Could you check a few things on this model? Use its own coordinates, in mm. A direction names the side the tool comes from. Coordinates: 2 decimals unless noted, no trailing zeros. Write each loop counter-clockwise with the first axis right and the second up, starting at its lowest first coordinate (ties: lowest second). Pieces come first, ordered by that corner, then holes. Notation, with made-up numbers: M 28.5,-16 L 45.5,-16 A25 cw 45.5,18 Z; hole C -2,-3.75 d6. An arc over 180 degrees is marked long. Write item = value, one per line.
```python
from build123d import *

# Parameters (mm, degrees)
F0_R     = 11.0236
F1_DEPTH = 6.35


with BuildPart() as f1:
    # F0 (on Front) → F1 (new body)
    with BuildSketch(Plane.XZ):
        with BuildLine():
            ThreePointArc((0.3274680596, -14.2837467396), (10.2179096725, -9.9863395783), (14.2875, 0))
            ThreePointArc((14.2875, 0), (13.8765823163, 3.4019287867), (12.6674657785, 6.6081742563))
            ThreePointArc((12.6674657785, 6.6081742563), (12.3386048381, 7.157527699), (12.0249856082, 7.7157227382))
            ThreePointArc((12.0249856082, 7.7157227382), (-0.0794118424, 14.2872793075), (-12.1100113559, 7.581575114))
            ThreePointArc((-12.1100113559, 7.581575114), (-12.3736819292, 7.1101281538), (-12.6482244827, 6.6449284184))
            ThreePointArc((-12.6482244827, 6.6449284184), (-12.2974900055, -7.2735408032), (-0.2689126433, -14.2849691018))
            ThreePointArc((-0.2689126433, -14.2849691018), (0.0292737936, -14.2824480224), (0.3274680596, -14.2837467396))
        make_face()
        Circle(F0_R, mode=Mode.SUBTRACT)
        with BuildLine():
            ThreePointArc((12.6674657785, 6.6081742563), (13.8765823163, 3.4019287867), (14.2875, 0))
            ThreePointArc((14.2875, 0), (10.2179096725, -9.9863395783), (0.3274680596, -14.2837467396))
            ThreePointArc((0.3274680596, -14.2837467396), (10.9182683676, -16.9609416049), (19.1217645686, -24.1744756619))
            Line((19.1217645686, -24.1744756619), (14.2986624039, -15.99905024))
            Line((14.2986624039, -15.99905024), (20.7900538279, -4.5075300019))
            Line((20.7900538279, -4.5075300019), (31.3741279928, -4.4080458119))
            ThreePointArc((31.3741279928, -4.4080458119), (20.6570695125, -1.2156835719), (12.6674657785, 6.6081742563))
        make_face()
        with BuildLine():
            ThreePointArc((12.0249856082, 7.7157227382), (12.3386048381, 7.157527699), (12.6674657785, 6.6081742563))
            ThreePointArc((12.6674657785, 6.6081742563), (12.3586388725, 7.1691492849), (12.0249856082, 7.7157227382))
        make_face()
        with BuildLine():
            ThreePointArc((-0.2689126433, -14.2849691018), (0.0292840868, -14.2874699892), (0.3274680596, -14.2837467396))
            ThreePointArc((0.3274680596, -14.2837467396), (0.0292737936, -14.2824480224), (-0.2689126433, -14.2849691018))
        make_face()
        with BuildLine():
            ThreePointArc((-12.1100113559, 7.581575114), (-0.0794118424, 14.2872793075), (12.0249856082, 7.7157227382))
            ThreePointArc((12.0249856082, 7.7157227382), (9.2100112148, 18.0768557667), (11.3474304636, 28.5986710771))
            Line((11.3474304636, 28.5986710771), (6.7062527423, 20.3825300019))
            Line((6.7062527423, 20.3825300019), (-6.4913914239, 20.258479762))
            Line((-6.4913914239, 20.258479762), (-11.8801477461, 29.3927203242))
            ThreePointArc((-11.8801477461, 29.3927203242), (-9.2812144735, 18.4585467989), (-12.1100113559, 7.581575114))
        make_face()
        with BuildLine():
            ThreePointArc((33.9876979941, -4.383479762), (32.6812582501, -4.4324944701), (31.3741279928, -4.4080458119))
            Line((31.3741279928, -4.4080458119), (20.7900538279, -4.5075300019))
            Line((20.7900538279, -4.5075300019), (14.2986624039, -15.99905024))
            Line((14.2986624039, -15.99905024), (19.1217645686, -24.1744756619))
            ThreePointArc((19.1217645686, -24.1744756619), (20.1269642499, -25.7329626623), (21.0049151462, -27.366520238))
            Line((21.0049151462, -27.366520238), (34.2025593124, -27.2424699981))
            Line((34.2025593124, -27.2424699981), (40.6939507364, -15.75094976))
            Line((40.6939507364, -15.75094976), (33.9876979941, -4.383479762))
        make_face()
        Polygon((22.5339984594, -24.6596288042), (17.4074408075, -15.9698295168), (22.3697489183, -7.1852007126), (32.4586146809, -7.0903711958), (37.5851723328, -15.7801704832), (32.622864222, -24.5647992874), align=None, mode=Mode.SUBTRACT)
        with BuildLine():
            Line((33.9876979941, -4.383479762), (31.3741279928, -4.4080458119))
            ThreePointArc((31.3741279928, -4.4080458119), (32.6812582501, -4.4324944701), (33.9876979941, -4.383479762))
        make_face()
        with BuildLine():
            ThreePointArc((-19.5323350277, -25.0159672189), (-11.251794814, -17.2249549892), (-0.2689126433, -14.2849691018))
            ThreePointArc((-0.2689126433, -14.2849691018), (-12.2974900055, -7.2735408032), (-12.6482244827, 6.6449284184))
            ThreePointArc((-12.6482244827, 6.6449284184), (-20.2295725455, -1.03712802), (-30.4613844896, -4.4723651173))
            Line((-30.4613844896, -4.4723651173), (-21.0049151462, -4.383479762))
            Line((-21.0049151462, -4.383479762), (-14.2986624039, -15.75094976))
            Line((-14.2986624039, -15.75094976), (-19.5323350277, -25.0159672189))
        make_face()
        with BuildLine():
            ThreePointArc((21.0049151462, -27.366520238), (20.1269642499, -25.7329626623), (19.1217645686, -24.1744756619))
            Line((19.1217645686, -24.1744756619), (21.0049151462, -27.366520238))
        make_face()
        with BuildLine():
            ThreePointArc((-12.6482244827, 6.6449284184), (-12.3736819292, 7.1101281538), (-12.1100113559, 7.581575114))
            ThreePointArc((-12.1100113559, 7.581575114), (-12.3879734912, 7.1183403285), (-12.6482244827, 6.6449284184))
        make_face()
        with BuildLine():
            ThreePointArc((13.1976441662, 31.87405024), (12.2062266956, 30.2738185559), (11.3474304636, 28.5986710771))
            Line((11.3474304636, 28.5986710771), (13.1976441662, 31.87405024))
        make_face()
        with BuildLine():
            Line((6.7062527423, 20.3825300019), (11.3474304636, 28.5986710771))
            ThreePointArc((11.3474304636, 28.5986710771), (12.2062266956, 30.2738185559), (13.1976441662, 31.87405024))
            Line((13.1976441662, 31.87405024), (6.4913914239, 43.241520238))
            Line((6.4913914239, 43.241520238), (-6.7062527423, 43.1174699981))
            Line((-6.7062527423, 43.1174699981), (-13.1976441662, 31.62594976))
            ThreePointArc((-13.1976441662, 31.62594976), (-12.5077667223, 30.5276997715), (-11.8801477461, 29.3927203242))
            Line((-11.8801477461, 29.3927203242), (-6.4913914239, 20.258479762))
            Line((-6.4913914239, 20.258479762), (6.7062527423, 20.3825300019))
        make_face()
        Polygon((-4.9623081108, 22.9653711958), (-10.0888657626, 31.6551704832), (-5.1265576519, 40.4397992874), (4.9623081108, 40.5346288042), (10.0888657626, 31.8448295168), (5.1265576519, 23.0602007126), align=None, mode=Mode.SUBTRACT)
        with BuildLine():
            ThreePointArc((-20.7900538279, -27.2424699981), (-20.1917898783, -26.1119356867), (-19.5323350277, -25.0159672189))
            Line((-19.5323350277, -25.0159672189), (-14.2986624039, -15.75094976))
            Line((-14.2986624039, -15.75094976), (-21.0049151462, -4.383479762))
            Line((-21.0049151462, -4.383479762), (-30.4613844896, -4.4723651173))
            ThreePointArc((-30.4613844896, -4.4723651173), (-32.331264033, -4.5652572938), (-34.2025593124, -4.5075300019))
            Line((-34.2025593124, -4.5075300019), (-40.6939507364, -15.99905024))
            Line((-40.6939507364, -15.99905024), (-33.9876979941, -27.366520238))
            Line((-33.9876979941, -27.366520238), (-20.7900538279, -27.2424699981))
        make_face()
        Polygon((-32.622864222, -7.1852007126), (-22.5339984594, -7.0903711958), (-17.4074408075, -15.7801704832), (-22.3697489183, -24.5647992874), (-32.4586146809, -24.6596288042), (-37.5851723328, -15.9698295168), align=None, mode=Mode.SUBTRACT)
        with BuildLine():
            Line((-20.7900538279, -27.2424699981), (-19.5323350277, -25.0159672189))
            ThreePointArc((-19.5323350277, -25.0159672189), (-20.1917898783, -26.1119356867), (-20.7900538279, -27.2424699981))
        make_face()
        with BuildLine():
            Line((-13.1976441662, 31.62594976), (-11.8801477461, 29.3927203242))
            ThreePointArc((-11.8801477461, 29.3927203242), (-12.5077667223, 30.5276997715), (-13.1976441662, 31.62594976))
        make_face()
        with BuildLine():
            ThreePointArc((-34.2025593124, -4.5075300019), (-32.331264033, -4.5652572938), (-30.4613844896, -4.4723651173))
            Line((-30.4613844896, -4.4723651173), (-34.2025593124, -4.5075300019))
        make_face()
    extrude(amount=F1_DEPTH)


solid = f1.part
```
Item 1: Imagine slicing it at C-C (y = -4.25). State how many separate pieces and enclosed holes the cut face has, and give its area (3 significant figures).
Numbers:
separate_pieces = 1
enclosed_holes = 4
area = 1,300 mm²
Item 2: For faces 5 (the face through (-7.64, -3.13, 35.99)), 6 (the face through (10.8, -3.1, -16.9)), 7 (the face through (-12.548, -3.131, 30.525)), which set-ups out of +Z, -Z, +X, -X, +Y, -Y let a thin tool reach every point of the face, with its end or its side?
Numbers:
face_5 = +Y, -Y
face_6 = -Z, +Y, -Y
face_7 = -X, +Y, -Y
Item 3: Imagine slicing it at D-D (z = 16). Write out the boundary of the cut face in (x, y).
Numbers:
outline = M -9.44,-6.35 L 9.37,-6.35 L 9.37,0 L -9.44,0 Z
Item 4: Imagine slicing it at A-A (z = 0). Write out the boundary of the cut face in (x, y), and give its area (3 significant figures).
Numbers:
outline = M -18.71,-6.35 L -11.02,-6.35 L -11.02,0 L -18.71,0 Z; M 11.02,-6.35 L 18.8,-6.35 L 18.8,0 L 11.02,0 Z
area = 98.2 mm²
Item 5: Imagine slicing it at B-B (x = -31.5). Write out the boundary of the cut face in (y, z).
Numbers:
outline = M -6.35,-27.34 L 0,-27.34 L 0,-24.65 L -6.35,-24.65 Z; M -6.35,-7.17 L 0,-7.17 L 0,-4.48 L -6.35,-4.48 Z
Item 6: If I drill on line 1 along Z through (x, y) = (0, -3.75); line 2 along X through (y, z) = (-3.25, -9); line 3 along X through (y, z) = (-5.75, 9), over which ranges is the centre line in solid material (lowest first)?
Numbers:
line_1 = -14.29 to -11.02, 11.02 to 23.01, 40.49 to 43.18
line_2 = -36.74 to -33.65, -21.41 to -6.37, 6.37 to 21.34, 33.59 to 36.71
line_3 = -11.4 to -6.37, 6.37 to 11.38
Item 7: If we mould it in two halves opening along Z, with no side actions, what happens to faces 1 (the face through (-20.17, -3.131, -26.145)), 2 (the face through (7.49, -3.13, 36.25)), 3 (the face through (12.26, -3.131, 30.213)), 4 (the face through (-37.4, -3.13, -10.17))? For each: pulls with the +Z half, pulls with the -Z half, needs draft (parallel to the pull), parting line crosses it, or undercut.
Numbers:
face_1 = pulls with the -Z half
face_2 = undercut
face_3 = undercut
face_4 = pulls with the +Z half
Item 8: I'm going to push a flat-ended pin straight in: P1, Ø2, axis at y = -3, z = 33, coming from the +X side. Where does the tip first touch, or does it pass through?
Numbers:
P1 = 13.12
